Input: part model. Units: mm. Frame: model coordinates. Give positions to 0.01 mm unless a question says otherwise; leave off trailing zeros. Loops run counter-clockwise (first coordinate to the right, second up) from the corner with the lowest first, then second, coordinate; pieces in that order, holes last. Notation, with made-up numbers: M 25,-25.5 L 60,-25.5 A19 ccw 60,0.5 Z; hole C 12,77.5 d5. An arc over 180 degrees is marked long. Answer as a JSON object with one key per item and string values. Group by question number.
1) Ray query, L1, parallel to X at y = 118, z = 0.6; L2, parallel to Y at x = 617, z = 0.25. Return the intervals inside material, ascending.
2) Section query C-C on x = 585.5. Return loops of the section in (y, z).
3) Section query B-B on z = 0.25. Return loops of the section in (x, y), plus the area to 3 significant figures.
4) Section query A-A on y = 72. Return loops of the section in (x, z).
5) First-contact query: P1, Ø8, axis at x = 231.5, y = 62.5, coming from the -Z side. Flat tip, straight axial feed; report the tip coordinate or a pass-through.
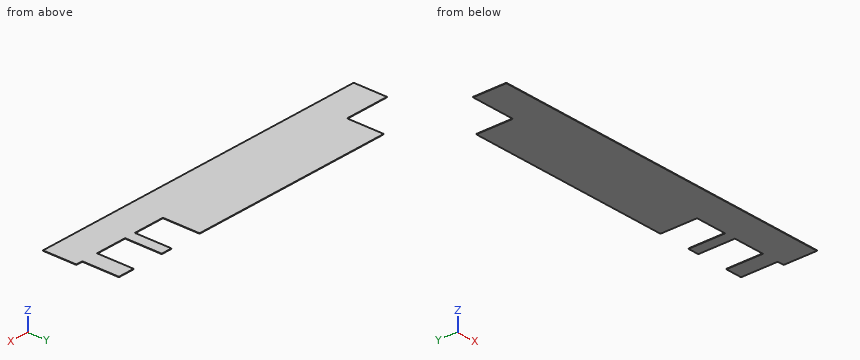
from build123d import *

# Parameters (mm, degrees)
F0_W     = 396.24
F0_H     = 69.85
F0_W_2   = 21.082
F0_W_3   = 31.75
F1_DEPTH = 0.8128


with BuildPart() as f1:
    # F0 (on Top) → F1 (new body)
    with BuildSketch(Plane.XY):
        Polygon((0, 63.5), (0, 0), (668.3375, 0), (668.3375, 63.5), (655.6375, 63.5), (623.8875, 63.5), (563.5625, 63.5), (542.4805, 63.5), (482.1555, 63.5), (85.9155, 63.5), align=None)
        with Locations((284.0355, 98.425)):
            Rectangle(F0_W, F0_H)
        with Locations((553.0215, 98.425)):
            Rectangle(F0_W_2, F0_H)
        with Locations((639.7625, 98.425)):
            Rectangle(F0_W_3, F0_H)
    extrude(amount=F1_DEPTH)


solid = f1.part
Output:
{
 "1": {"L1": "x = 85.92 to 482.16, 542.48 to 563.56, 623.89 to 655.64", "L2": "y = 0 to 63.5"},
 "2": {"outline": "M 0,0 L 63.5,0 L 63.5,0.81 L 0,0.81 Z"},
 "3": {"outline": "M 0,0 L 668.34,0 L 668.34,63.5 L 655.64,63.5 L 655.64,133.35 L 623.89,133.35 L 623.89,63.5 L 563.56,63.5 L 563.56,133.35 L 542.48,133.35 L 542.48,63.5 L 482.16,63.5 L 482.16,133.35 L 85.92,133.35 L 85.92,63.5 L 0,63.5 Z", "area": "73,800 mm^2"},
 "4": {"outline": "M 85.92,0 L 482.16,0 L 482.16,0.81 L 85.92,0.81 Z; M 542.48,0 L 563.56,0 L 563.56,0.81 L 542.48,0.81 Z; M 623.89,0 L 655.64,0 L 655.64,0.81 L 623.89,0.81 Z"},
 "5": {"P1": "stops at z = 0"}
}
